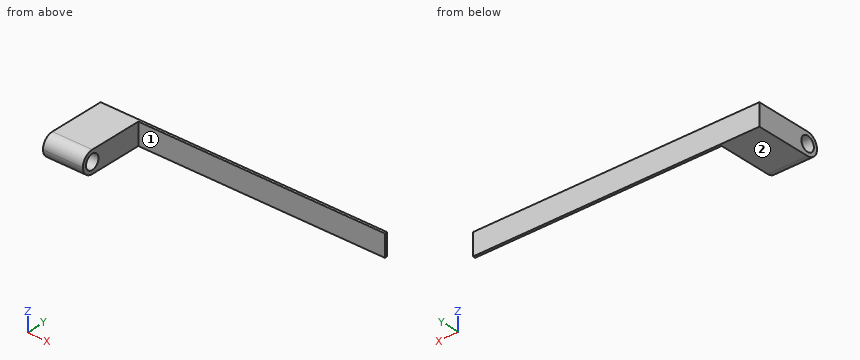
from build123d import *

# Parameters (mm, degrees)
F0_W      = 279.4
F0_H      = 330.2
F1_DEPTH  = 152.4
F3_D      = 101.6
F5_DEPTH  = 279.4
F7_DEPTH  = 137.7526689321
F8_W      = 17.7074246799
F8_H      = 152.4
F9_DEPTH  = 1397
F11_DEPTH = 330.2


with BuildPart() as f1:
    # F0 (on Top) → F1 (new body)
    with BuildSketch(Plane.XY):
        with Locations((15.0600075722, 36.8478087073)):
            Rectangle(F0_W, F0_H)
    extrude(amount=F1_DEPTH)

    # F3 (through all)
    with Locations(Plane.YZ.offset(154.7600075722)):
        with Locations((-52.0521912927, 76.2)):
            Hole(F3_D / 2)

    # F4 (on face) → F5 (cut)
    with BuildSketch(Plane(origin=(-124.6399924278, 0, 0), x_dir=(0, -1, 0), z_dir=(-1, 0, 0))):
        with BuildLine():
            ThreePointArc((128.2521912927, 76.2), (105.9337280192, 22.3184632736), (52.0521912927, 0))
            Line((52.0521912927, 0), (65.0011226535, 0))
            Line((65.0011226535, 0), (128.2521912927, 0))
            Line((128.2521912927, 0), (128.2521912927, 76.2))
        make_face()
        with BuildLine():
            ThreePointArc((52.0521912927, 152.4), (105.9337280192, 130.0815367264), (128.2521912927, 76.2))
            Line((128.2521912927, 76.2), (128.2521912927, 152.4))
            Line((128.2521912927, 152.4), (65.0011226535, 152.4))
            Line((65.0011226535, 152.4), (52.0521912927, 152.4))
        make_face()
    extrude(amount=-F5_DEPTH, mode=Mode.SUBTRACT)

    # F7 (add): a face of the model
    f7_faces = [f1.faces().sort_by_distance(p)[0] for p in [
        (15.0600075722, 201.9478087073, 76.2),
    ]]
    extrude(f7_faces, amount=F7_DEPTH)

    # F8 (on face) → F9 (join)
    with BuildSketch(Plane.YZ.offset(154.7600075722)):
        with Locations((330.8467652994, 76.2)):
            Rectangle(F8_W, F8_H)
    extrude(amount=F9_DEPTH)

    # F11 (add): a face of the model
    f11_faces = [f1.faces().sort_by_distance(p)[0] for p in [
        (1551.7600075722, 330.8467652994, 76.2),
    ]]
    extrude(f11_faces, amount=F11_DEPTH)


solid = f1.part
Part model, mm, in its own coordinate system. Face numbers are marked on the shaded views. A direction names the side the tool comes from. Coordinates: 2 decimals unless noted, no trailing zeros. Loops run counter-clockwise (first coordinate to the right, second up) from the corner with the lowest first, then second, coordinate; pieces in that order, holes last. Notation, with made-up numbers: M 77,14 L 84,14 A27 cw 84,47 Z; hole C 76.5,-11.75 d10. An arc over 180 degrees is marked long. Use a Markdown table: item, result. Add a question column.
Q1. Cut at C-C (y = 47). Write the cut outline in (x, z).
Q2. Cut at B-B (x = 685). Write the cut outline in (y, z), and give its area (3 significant figures).
Q3. Probe L1, parallel to Y at x = -60, z = 76; L2, parallel to X at y = 187.5, z = 33.5; L3, parallel to Y at x = 1400, z = 54.5. List the from-to ranges inside material, lowest first.
Q4. Pin check, flat tips, straight feed: P1, Ø5, axis at x = 920, z = 126.5, coming from the -Y side; P2, Ø2, axis at y = 94, z = 115, coming from the +X side. Stop position of each tip, or through.
Q5. Which spindle directions (+Z, -Z, +X, -X, +Y, -Y) get a long thin tool onto all of the face, cutting with end or side? Do the marked faces 1 and 2. Say none if no direction does.
Q6. Cut at A-A (z = 94). Write the cut outline in (x, y).
Worked out:
| question | item | result |
|---|---|---|
| 1 | outline | M -124.64,0 L 154.76,0 L 154.76,152.4 L -124.64,152.4 Z |
| 2 | outline | M 321.99,0 L 339.7,0 L 339.7,152.4 L 321.99,152.4 Z |
| 2 | area | 2,700 mm2 |
| 3 | L1 | y = -128.25 to -102.85, -1.25 to 339.7 |
| 3 | L2 | x = -124.64 to 154.76 |
| 3 | L3 | y = 321.99 to 339.7 |
| 4 | P1 | stops at y = 321.99 |
| 4 | P2 | stops at x = 154.76 |
| 5 | face 1 | +Z, -Z, +X, -Y |
| 5 | face 2 | -Z, +X, -X, +Y, -Y |
| 6 | outline | M -124.64,-126.14 L 154.76,-126.14 L 154.76,-99.63 L -124.64,-99.63 Z; M -124.64,-4.47 L 154.76,-4.47 L 154.76,321.99 L 1881.96,321.99 L 1881.96,339.7 L -124.64,339.7 Z |
